from build123d import *

# Parameters (mm, degrees)
F0_R     = 1.6002
F0_R_2   = 2.3749
F1_DEPTH = 1.89738


with BuildPart() as f1:
    # F0 (on Front) → F1 (new body)
    with BuildSketch(Plane.XZ):
        with BuildLine():
            Line((30.803165, 27.752104), (-7.296835, 27.752104))
            Line((-7.296835, 27.752104), (-7.240266, 18.437498))
            ThreePointArc((-7.240266, 18.437498), (-6.286852, 16.216634), (-4.046344, 15.310343))
            Line((-4.046344, 15.310343), (-0.869708, 15.329635))
            Line((-0.869708, 15.329635), (24.528914, 15.279349))
            Line((24.528914, 15.279349), (27.703914, 15.279349))
            ThreePointArc((27.703914, 15.279349), (29.943251, 16.222922), (30.859515, 18.473572))
            Line((30.859515, 18.473572), (30.803165, 27.752104))
        make_face()
        with Locations((-4.519141, 18.598825)):
            Circle(F0_R, mode=Mode.SUBTRACT)
        with Locations((28.207415, 18.36364)):
            Circle(F0_R, mode=Mode.SUBTRACT)
        with Locations((-4.121835, 24.740549)):
            Circle(F0_R_2, mode=Mode.SUBTRACT)
        with Locations((27.628165, 24.740549)):
            Circle(F0_R_2, mode=Mode.SUBTRACT)
    extrude(amount=F1_DEPTH)


solid = f1.part
The model under review builds one solid part; all positions refer to its coordinate system, in mm. Round coordinates to 2 decimals unless told otherwise and drop trailing zeros. Loops run counter-clockwise (first coordinate to the right, second up) from the corner with the lowest first, then second, coordinate; pieces in that order, holes last. Notation, with made-up numbers: (-36.5, 3) -> (-1.5, 3) arc R18 ccw to (-1.5, 38) -> close; hole circle Ø1 at (-13.75, 61.5). An arc over 180 degrees is marked (long way). One line per question, with ' | ' between items. Start each with the question number.
Item 1: For pin 1 (1 mm diameter, centred on x = 16, y = -1, fed in from -Z), flat-tipped, find the tip position at first contact; note if it passes through.
Item 2: Draft analysis for pull direction X (two halves, no side actions). For faces 1 (the face through (12, -1.897, 22)), 2 (the face through (29.92, -0.94, 16.2)), 3 (the face through (-4.4, -0.9, 27.1)), 4 (the face through (26.94, -0.94, 17.39)), state which applies: +X half, -X half, draft (parallel to the pull), parting line (faces both ways), or undercut.
Item 3: Add section B-B, the plane y = -0.4. Count the separate pieces of the cut face and the enclosed holes in it, then the cut area to 3 significant figures.
Item 4: Add section A-A, the plane z = 26.5. Write out the cut boundary in (x, y).
Item 5: Wall thickness on line 1 along X through (y, z) = (-1, 18.5); line 2 along X through (y, z) = (-1.6, 25.25); line 3 along Z through (x, y) = (20, -0.95): over which ranges is each line inside the solid? List them lowest first. Write a range as [from, to].
Item 6: Add section C-C, the plane z = 23. Write out the cut boundary in (x, y).
Return value:
1) pin 1: stops at z = 15.3
2) face 1: draft | face 2: +X half | face 3: undercut | face 4: undercut
3) separate pieces: 1 | enclosed holes: 4 | area: 418 mm2
4) outline: (-7.29, -1.9) -> (-5.72, -1.9) -> (-5.72, 0) -> (-7.29, 0) -> close; (-2.53, -1.9) -> (26.03, -1.9) -> (26.03, 0) -> (-2.53, 0) -> close; (29.22, -1.9) -> (30.81, -1.9) -> (30.81, 0) -> (29.22, 0) -> close
5) line 1: x = [-7.24, -6.12], [-2.92, 26.61], [29.8, 30.86] | line 2: x = [-7.28, -6.44], [-1.8, 25.31], [29.95, 30.82] | line 3: z = [15.29, 27.75]
6) outline: (-7.27, -1.9) -> (-5.74, -1.9) -> (-5.74, 0) -> (-7.27, 0) -> close; (-2.51, -1.9) -> (26.01, -1.9) -> (26.01, 0) -> (-2.51, 0) -> close; (29.24, -1.9) -> (30.83, -1.9) -> (30.83, 0) -> (29.24, 0) -> close
